```python
from build123d import *

# Parameters (mm, degrees)
EXTRUDE3_DEPTH = 15.24
EXTRUDE4_DEPTH = 6.477
SKETCH7_R      = 7.8994
EXTRUDE5_DEPTH = 4.0132
SKETCH8_R      = 2.2987
EXTRUDE6_DEPTH = 4.2926
SKETCH9_R      = 4.4196
EXTRUDE7_DEPTH = 4.4196
SKETCH12_R     = 1.179287719
SKETCH12_R_2   = 1.905
SKETCH12_R_3   = 4.7244
EXTRUDE8_DEPTH = 19.177


with BuildPart() as part:
    # Sketch4 → Extrude3 (new body)
    with BuildSketch(Plane.XY):
        with BuildLine():
            Line((-34.989977361, 16.714860485), (-26.837942516, 16.714860485))
            ThreePointArc((-26.837942516, 16.714860485), (-25.910547148, 16.539503762), (-25.11120297, 16.037646178))
            Line((-25.11120297, 16.037646178), (-20.513533707, 11.775761749))
            ThreePointArc((-20.513533707, 11.775761749), (-19.714189529, 11.273904165), (-18.786794161, 11.098547442))
            Line((-18.786794161, 11.098547442), (16.238704516, 11.098547442))
            ThreePointArc((16.238704516, 11.098547442), (17.210720434, 11.291893429), (18.03475574, 11.842496218))
            Line((18.03475574, 11.842496218), (22.163171231, 15.970911709))
            ThreePointArc((22.163171231, 15.970911709), (22.987206537, 16.521514497), (23.959222455, 16.714860485))
            Line((23.959222455, 16.714860485), (48.342712132, 16.714860485))
            ThreePointArc((48.342712132, 16.714860485), (50.138763356, 15.970911709), (50.882712132, 14.174860485))
            Line((50.882712132, 14.174860485), (50.882712132, -10.580714332))
            ThreePointArc((50.882712132, -10.580714332), (51.626660908, -12.376765556), (53.422712132, -13.120714332))
            Line((53.422712132, -13.120714332), (60.311539532, -13.120714332))
            Line((60.311539532, -13.120714332), (60.311539532, -19.76149571))
            Line((60.311539532, -19.76149571), (32.406215876, -19.76149571))
            ThreePointArc((32.406215876, -19.76149571), (31.669198311, -19.652216819), (30.995598433, -19.333783198))
            Line((30.995598433, -19.333783198), (18.568386733, -11.034703794))
            ThreePointArc((18.568386733, -11.034703794), (17.894786855, -10.716270173), (17.157769291, -10.606991282))
            Line((17.157769291, -10.606991282), (-17.723220352, -10.606991282))
            ThreePointArc((-17.723220352, -10.606991282), (-19.519271576, -11.350940058), (-20.263220352, -13.146991282))
            Line((-20.263220352, -13.146991282), (-20.263220352, -19.76149571))
            Line((-20.263220352, -19.76149571), (-35.4927874, -19.76149571))
            Line((-35.4927874, -19.76149571), (-35.4927874, -13.120714332))
            Line((-35.4927874, -13.120714332), (-28.163499743, -13.120714332))
            Line((-28.163499743, -13.120714332), (-28.163499743, -4.013214075))
            ThreePointArc((-28.163499743, -4.013214075), (-28.907448519, -2.217162851), (-30.703499743, -1.473214075))
            Line((-30.703499743, -1.473214075), (-34.989977361, -1.473214075))
            ThreePointArc((-34.989977361, -1.473214075), (-36.786028585, -0.729265299), (-37.529977361, 1.066785925))
            Line((-37.529977361, 1.066785925), (-37.529977361, 14.174860485))
            ThreePointArc((-37.529977361, 14.174860485), (-36.786028585, 15.970911709), (-34.989977361, 16.714860485))
        make_face()
    extrude(amount=-EXTRUDE3_DEPTH)

    # Sketch1 → Extrude4 (cut)
    with BuildSketch(Plane.XY):
        with BuildLine():
            ThreePointArc((19.458991626, 4.314801956), (12.038580445, 8.580199555), (4.913681626, 3.837633204))
            ThreePointArc((4.913681626, 3.837633204), (-2.477718374, 8.584569756), (-9.869118374, 3.837633204))
            ThreePointArc((-9.869118374, 3.837633204), (-15.272484602, 8.337693135), (-22.163825334, 6.939004858))
            ThreePointArc((-22.163825334, 6.939004858), (-33.125915624, 9.855374055), (-25.30153955, 1.642471287))
            ThreePointArc((-25.30153955, 1.642471287), (-19.566986279, -7.337311806), (-9.869118374, -2.924493692))
            ThreePointArc((-9.869118374, -2.924493692), (-2.477718374, -7.671430244), (4.913681626, -2.924493692))
            ThreePointArc((4.913681626, -2.924493692), (12.038580445, -7.667060044), (19.458991626, -3.401662445))
            ThreePointArc((19.458991626, -3.401662445), (47.839681626, 0.456569756), (19.458991626, 4.314801956))
        make_face()
    extrude(amount=-EXTRUDE4_DEPTH, mode=Mode.SUBTRACT)

    # Sketch7 → Extrude5 (cut)
    with BuildSketch(Plane.XY.offset(-6.477)):
        with Locations((33.387081626, 0.456569756)):
            Circle(SKETCH7_R)
    extrude(amount=-EXTRUDE5_DEPTH, mode=Mode.SUBTRACT)

    # Sketch8 → Extrude6 (cut)
    with BuildSketch(Plane.XY.offset(-6.477)):
        with Locations((12.305081626, 0.456569756)):
            Circle(SKETCH8_R)
        with Locations((-2.477718374, 0.456569756)):
            Circle(SKETCH8_R)
        with Locations((-17.260518374, 0.456569756)):
            Circle(SKETCH8_R)
    extrude(amount=-EXTRUDE6_DEPTH, mode=Mode.SUBTRACT)

    # Sketch9 → Extrude7 (cut)
    with BuildSketch(Plane.XY.offset(-6.477)):
        with Locations((-28.055981517, 6.851899403)):
            Circle(SKETCH9_R)
    extrude(amount=-EXTRUDE7_DEPTH, mode=Mode.SUBTRACT)

    # Sketch12 → Extrude8 (cut, symmetric)
    with BuildSketch(Plane.XY):
        with Locations((-28.055981517, 6.851899403)):
            Circle(SKETCH12_R)
        with Locations((-24.233740004, -13.623099256)):
            Circle(SKETCH12_R_2)
        with Locations((47.080626595, -13.623099256)):
            Circle(SKETCH12_R_2)
        with Locations((47.080626595, 13.774579835)):
            Circle(SKETCH12_R_2)
        with Locations((33.387081626, 0.456569756)):
            Circle(SKETCH12_R_3)
        with Locations((4.913681626, -7.85150728)):
            Circle(SKETCH12_R_2)
        with Locations((4.913681626, 8.764646791)):
            Circle(SKETCH12_R_2)
        with Locations((-34.554939326, 13.665214221)):
            Circle(SKETCH12_R_2)
    extrude(amount=EXTRUDE8_DEPTH, both=True, mode=Mode.SUBTRACT)


solid = part.part
```
Here's how the part is built. I have some questions about the finished solid (model axes, mm). A direction names the side the tool comes from. Give positions to 0.01 mm unless a question says otherwise; leave off trailing zeros. Loops run counter-clockwise (first coordinate to the right, second up) from the corner with the lowest first, then second, coordinate; pieces in that order, holes last. Notation, with made-up numbers: M 56.25,-39.75 L 105.25,-39.75 A17 ccw 105.25,-17.75 Z; hole C -33,-8.5 d5. An arc over 180 degrees is marked long. Return JSON: item names as keys, results as strings.
Item 1: I'm going to push flat-ended pins straight in: pin 1 Ø2.5 at (x, y) = (-18, 1) entering from +Z; pin 2 Ø6 at (x, z) = (-7.5, -13) entering from +Y; pin 3 Ø12.5 at (x, y) = (37, -2.5) entering from +Z. Where does each tip first touch, or does it pass through?
A:
{"pin 1": "stops at z = -10.77", "pin 2": "stops at y = 11.1", "pin 3": "stops at z = -6.48"}
Item 2: Imagine slicing it at A-A on x = -8.5. List the corners of the cut face in (y, z) for me.
A:
{"outline": "M -10.61,-15.24 L 11.1,-15.24 L 11.1,0 L 5.92,0 L 5.92,-6.48 L -5,-6.48 L -5,0 L -10.61,0 Z"}
Item 3: Thinking about a two-plate mould opening in X: for faces 1 (the cylindrical face through (-28.888, -2.237, -7.513)), 2 (the cylindrical face through (-19.73, 11.28, -7.51)), 3 (the flat face through (57, -13.121, -8)), which applies, released by +X, released by -X, zero draft, split by the parting line, or undercut?
A:
{"face 1": "released by -X", "face 2": "undercut", "face 3": "zero draft"}
Item 4: Imagine slicing it at B-B on z = -7.75. State how many separate pieces and enclosed holes the cut face has, then the cut area to 3 significant figures.
A:
{"separate pieces": "1", "enclosed holes": "11", "area": "2,140 mm^2"}
Item 5: On a 3-axis mill with a long thin cutter (end or side, diameter ignored), from which of +Z, -Z, +X, -X, +Y, -Y can I reach the whole of each face in a straight line? I mean faces 4 (the cylindrical face through (-19.5, -11.33, -7.51)), 5 (the flat face through (-2, 11.099, -8)), 6 (the cylindrical face through (10.48, -0.94, -8.59)). Say none if no direction works.
A:
{"face 4": "+Z, -Z, -Y", "face 5": "+Z, -Z, +Y", "face 6": "+Z"}
Item 6: Please list where these lines run through material, in increasing order: line 1 (Y direction, x = 33.5, z = -12.5); line 2 (Y direction, x = 48.5, z = -9); line 3 (X direction, y = -4, z = -5.75).
A:
{"line 1": "y = -19.76 to -4.27, 5.18 to 16.71", "line 2": "y = -19.76 to -14.89, -12.35 to 12.5, 15.05 to 16.71", "line 3": "x = -28.16 to -24.06, -10.46 to -9.28, 4.32 to 5.51, 19.1 to 19.64, 47.14 to 50.88"}
